```python
from build123d import *

# Parameters (mm, degrees)
SKETCH1_W               = 50
SKETCH1_H               = 50
BOSS_EXTRUDE1_DEPTH     = 2
CUT_EXTRUDE1_DEPTH      = 36.411862419
CUT_EXTRUDE1_DEPTH_BACK = 36.411862419
SKETCH2_W               = 2.3
SKETCH2_H               = 16
SKETCH3_W               = 22
SKETCH3_H               = 3
SKETCH3_W_2             = 5
BOSS_EXTRUDE2_DEPTH     = 14.5
SKETCH4_W               = 5
SKETCH4_H               = 2
SKETCH4_W_2             = 4
BOSS_EXTRUDE11_DEPTH    = 13
SKETCH5_W               = 3.5
SKETCH5_H               = 3
SKETCH5_W_2             = 18
BOSS_EXTRUDE12_DEPTH    = 1
SKETCH6_W               = 3.5
SKETCH6_H               = 12
SKETCH6_W_2             = 3
BOSS_EXTRUDE13_DEPTH    = 9
SKETCH7_W               = 3.5
SKETCH7_H               = 8
BOSS_EXTRUDE14_DEPTH    = 11
SKETCH8_W               = 2
SKETCH8_H               = 8
BOSS_EXTRUDE15_DEPTH    = 8
BOSS_EXTRUDE16_DEPTH    = 20
SKETCH10_W              = 2
SKETCH10_H              = 15
BOSS_EXTRUDE17_DEPTH    = 8
FILLET1_R               = 10
FILLET2_START           = -18
FILLET2_DEPTH           = 0.13972
FILLET2_START_2         = -17.86028
FILLET2_2_DEPTH         = 8.733515347
FILLET2_START_3         = -25
FILLET2_3_DEPTH         = 8.873235347
CUT_EXTRUDE2_DEPTH      = 50.964612469
CUT_EXTRUDE2_DEPTH_BACK = 50.964612469
SKETCH11_R              = 1.65
SKETCH13_W              = 2.5
SKETCH13_H              = 21
BOSS_EXTRUDE18_DEPTH    = 2
FILLET3_R               = 4
SKETCH14_W              = 17.5
SKETCH14_H              = 3
BOSS_EXTRUDE19_DEPTH    = 19.5
FILLET4_R               = 3
SKETCH15_W              = 14.5
SKETCH15_H              = 2
BOSS_EXTRUDE20_DEPTH    = 3
FILLET5_R               = 3
FILLET6_R               = 3


with BuildPart() as part:
    # Sketch1 → Boss-Extrude1 (new body)
    with BuildSketch(Plane.XY):
        Rectangle(SKETCH1_W, SKETCH1_H)
    extrude(amount=BOSS_EXTRUDE1_DEPTH)

    # Sketch2 → Cut-Extrude1 (cut, two sides: drawn at the far end of the back side and taken through both)
    with BuildSketch(Plane.XY.offset(2).offset(-CUT_EXTRUDE1_DEPTH_BACK)):
        with Locations((-19.85, 5.5)):
            Rectangle(SKETCH2_W, SKETCH2_H)
        with Locations((22.95, 5.5)):
            Rectangle(SKETCH2_W, SKETCH2_H)
    extrude(amount=CUT_EXTRUDE1_DEPTH + CUT_EXTRUDE1_DEPTH_BACK, mode=Mode.SUBTRACT)

    # Sketch3 → Boss-Extrude2 (add)
    with BuildSketch(Plane(origin=(0, 0, 0), x_dir=(-1, 0, 0), z_dir=(0, 0, -1))):
        with Locations((-14, -21.5)):
            Rectangle(SKETCH3_W, SKETCH3_H)
        with Locations((22.5, -21.5)):
            Rectangle(SKETCH3_W_2, SKETCH3_H)
    extrude(amount=BOSS_EXTRUDE2_DEPTH)

    # Sketch4 → Boss-Extrude11 (add)
    with BuildSketch(Plane(origin=(0, 0, 0), x_dir=(-1, 0, 0), z_dir=(0, 0, -1))):
        with Locations((3.5, -24)):
            Rectangle(SKETCH4_W, SKETCH4_H)
        with Locations((13.5, -24)):
            Rectangle(SKETCH4_W_2, SKETCH4_H)
    extrude(amount=BOSS_EXTRUDE11_DEPTH)

    # Sketch5 → Boss-Extrude12 (add)
    with BuildSketch(Plane(origin=(0, 0, -14.5), x_dir=(-1, 0, 0), z_dir=(0, 0, -1))):
        with Locations((23.25, -21.5)):
            Rectangle(SKETCH5_W, SKETCH5_H)
        with Locations((-16, -21.5)):
            Rectangle(SKETCH5_W_2, SKETCH5_H)
    extrude(amount=BOSS_EXTRUDE12_DEPTH)

    # Sketch6 → Boss-Extrude13 (add)
    with BuildSketch(Plane(origin=(0, 0, 0), x_dir=(-1, 0, 0), z_dir=(0, 0, -1))):
        with Locations((23.25, -14)):
            Rectangle(SKETCH6_W, SKETCH6_H)
        with Locations((-23.5, -14)):
            Rectangle(SKETCH6_W_2, SKETCH6_H)
    extrude(amount=BOSS_EXTRUDE13_DEPTH)

    # Sketch7 → Boss-Extrude14 (add)
    with BuildSketch(Plane(origin=(0, 0, -9), x_dir=(-1, 0, 0), z_dir=(0, 0, -1))):
        with Locations((23.25, -14)):
            Rectangle(SKETCH7_W, SKETCH7_H)
    extrude(amount=BOSS_EXTRUDE14_DEPTH)

    # Sketch8 → Boss-Extrude15 (add)
    with BuildSketch(Plane.ZY.offset(25)):
        with Locations((-19, -14)):
            Rectangle(SKETCH8_W, SKETCH8_H)
    extrude(amount=BOSS_EXTRUDE15_DEPTH)

    # Sketch9 → Boss-Extrude16 (add)
    with BuildSketch(Plane(origin=(0, 0, 0), x_dir=(-1, 0, 0), z_dir=(0, 0, -1))):
        Polygon((11.748068925, 25), (11.748068925, 23), (23, 23), (23, 15.388525781), (25, 15.388525781), (25, 25), align=None)
    extrude(amount=BOSS_EXTRUDE16_DEPTH)

    # Sketch10 → Boss-Extrude17 (add)
    with BuildSketch(Plane.ZY.offset(25)):
        with Locations((-19, 22.888525781)):
            Rectangle(SKETCH10_W, SKETCH10_H)
    extrude(amount=BOSS_EXTRUDE17_DEPTH)

    # Fillet1
    # the kernel refuses this fillet: 10 mm, written as the material it adds along each edge
    with BuildSketch(Plane(origin=(-25, 25, -20), x_dir=(1, 0, 0), z_dir=(0, 0, 1))) as fillet1_piece_1:
        with BuildLine():
            CenterArc((8.873235347, 10), FILLET1_R, 207.461173358, 62.538826642)
            Line((0, 5.388525781), (0, 0))
            Line((0, 0), (8.873235347, 0))
        make_face()
    extrude(amount=2)

    # Fillet2: read off the stored shape, not the designer's step
    # Fillet2 outline → Fillet2 (add)
    with BuildSketch(Plane.XY.offset(FILLET2_START)):
        with BuildLine():
            Line((-25, 30.388525781), (-25, 25))
            Line((-25, 25), (-16.126764653, 25))
            ThreePointArc((-16.126764653, 25), (-21.317393604, 26.452639525), (-25, 30.388525781))
        make_face()
    extrude(amount=FILLET2_DEPTH)

    # Fillet2 2 outline → Fillet2 2 (add)
    with BuildSketch(Plane.XY.offset(FILLET2_START_2)):
        with BuildLine():
            Line((-25, 30.388525781), (-25, 25))
            Line((-25, 25), (-16.126764653, 25))
            ThreePointArc((-16.126764653, 25), (-21.317393604, 26.452639525), (-25, 30.388525781))
        make_face()
    extrude(amount=FILLET2_2_DEPTH)

    # Fillet2 3 outline → Fillet2 3 (cut)
    with BuildSketch(Plane.YZ.offset(FILLET2_START_3)):
        with BuildLine():
            ThreePointArc((25, -9.126764653), (26.452639525, -14.317393604), (30.388525781, -18))
            Line((30.388525781, -18), (32, -18.837492924))
            Line((32, -18.837492924), (32, -9.126764653))
            Line((32, -9.126764653), (25, -9.126764653))
        make_face()
    extrude(amount=FILLET2_3_DEPTH, mode=Mode.SUBTRACT)

    # Sketch11 → Cut-Extrude2 (cut, two sides: drawn at the far end of the back side and taken through both)
    with BuildSketch(Plane(origin=(0, 0, -20), x_dir=(-1, 0, 0), z_dir=(0, 0, -1)).offset(-CUT_EXTRUDE2_DEPTH_BACK)):
        with Locations((28.55, 26)):
            Circle(SKETCH11_R)
        with Locations((28.55, -14)):
            Circle(SKETCH11_R)
    extrude(amount=CUT_EXTRUDE2_DEPTH + CUT_EXTRUDE2_DEPTH_BACK, mode=Mode.SUBTRACT)

    # Sketch13 → Boss-Extrude18 (add)
    with BuildSketch(Plane(origin=(0, 0, 0), x_dir=(-1, 0, 0), z_dir=(0, 0, -1))):
        with Locations((-26.25, 5.5)):
            Rectangle(SKETCH13_W, SKETCH13_H)
    extrude(amount=-BOSS_EXTRUDE18_DEPTH)

    # Fillet3
    # the kernel refuses this fillet: 4 mm, written as the material it adds along each edge
    with BuildSketch(Plane(origin=(25, -5, -9.270248109), x_dir=(0, -1, 0), z_dir=(0, 0, 1))) as fillet3_piece_1_section:
        with BuildLine():
            CenterArc((3.708099244, 4), FILLET3_R, 202.024312837, 67.975687163)
            Line((0, 2.5), (-0.074161985, 2.47))
            ThreePointArc((-0.074161985, 2.47), (-0.08, 1.25), (-0.08, 0))
            Line((-0.08, 0), (0, -0.08))
            Line((0, -0.08), (3.708099244, -0.08))
            Line((3.708099244, -0.08), (3.708099244, 0))
        make_face()
    fillet3_piece_1 = extrude(amount=11.270248109, mode=Mode.PRIVATE)
    fillet3_piece_1 = split(fillet3_piece_1, bisect_by=Plane(origin=(25, -5, 0), z_dir=(0, 0, -1)), keep=Keep.TOP, mode=Mode.PRIVATE)
    fillet3_piece_1 = split(fillet3_piece_1, bisect_by=Plane(origin=(25, -8, -9.270248109), z_dir=(0, -1, 0)), keep=Keep.TOP, mode=Mode.PRIVATE)
    fillet3_piece_1 = split(fillet3_piece_1, bisect_by=Plane(origin=(25, -5, -9), z_dir=(0, 0, 1)), keep=Keep.TOP, mode=Mode.PRIVATE)
    add(fillet3_piece_1)
    with BuildSketch(Plane(origin=(25, -5, 0), x_dir=(0, -1, 0), z_dir=(0, 0, 1))) as fillet3_piece_2_section:
        with BuildLine():
            CenterArc((3.708099244, 4), FILLET3_R, 202.024312837, 67.975687163)
            Line((0, 2.5), (-0.074161985, 2.47))
            ThreePointArc((-0.074161985, 2.47), (-0.08, 1.25), (-0.08, 0))
            Line((-0.08, 0), (0, -0.08))
            Line((0, -0.08), (3.708099244, -0.08))
            Line((3.708099244, -0.08), (3.708099244, 0))
        make_face()
    fillet3_piece_2 = extrude(amount=2, mode=Mode.PRIVATE)
    fillet3_piece_2 = split(fillet3_piece_2, bisect_by=Plane(origin=(25, -8, 0), z_dir=(0, -1, 0)), keep=Keep.TOP, mode=Mode.PRIVATE)
    add(fillet3_piece_2)
    with BuildSketch(Plane(origin=(25, -5, 0), x_dir=(0, -1, 0), z_dir=(0, 0, 1))) as fillet3_piece_3_section:
        with BuildLine():
            CenterArc((3.708099244, 4), FILLET3_R, 202.024312837, 67.975687163)
            Line((0, 2.5), (-0.074161985, 2.47))
            ThreePointArc((-0.074161985, 2.47), (-0.08, 1.25), (-0.08, 0))
            Line((-0.08, 0), (0, -0.08))
            Line((0, -0.08), (3.708099244, -0.08))
            Line((3.708099244, -0.08), (3.708099244, 0))
        make_face()
    fillet3_piece_3 = extrude(amount=2, mode=Mode.PRIVATE)
    fillet3_piece_3 = split(fillet3_piece_3, bisect_by=Plane(origin=(25, -8, 0), z_dir=(0, 1, 0)), keep=Keep.TOP, mode=Mode.PRIVATE)
    add(fillet3_piece_3)
    with BuildSketch(Plane(origin=(25, 16, 0), x_dir=(0, 1, 0), z_dir=(0, 0, 1))) as fillet3_piece_4:
        with BuildLine():
            CenterArc((3.708099244, -4), FILLET3_R, 90, 67.975687163)
            Line((0, -2.5), (-0.074161985, -2.47))
            ThreePointArc((-0.074161985, -2.47), (-0.08, -1.25), (-0.08, 0))
            Line((-0.08, 0), (0, 0.08))
            Line((0, 0.08), (3.708099244, 0.08))
            Line((3.708099244, 0.08), (3.708099244, 0))
        make_face()
    extrude(amount=2)

    # Sketch14 → Boss-Extrude19 (add)
    with BuildSketch(Plane(origin=(0, 0, 0), x_dir=(-1, 0, 0), z_dir=(0, 0, -1))):
        with Locations((-13.25, -17.4)):
            Rectangle(SKETCH14_W, SKETCH14_H)
    extrude(amount=BOSS_EXTRUDE19_DEPTH)

    # Fillet4
    fillet4_edges = [part.edges().sort_by_distance(p)[0] for p in [
        (-3.5, -23, 0),
        (-13.5, -23, 0),
    ]]
    fillet(fillet4_edges, radius=FILLET4_R)

    # Sketch15 → Boss-Extrude20 (add)
    with BuildSketch(Plane.XZ.offset(25)):
        with Locations((-8.25, 1)):
            Rectangle(SKETCH15_W, SKETCH15_H)
    extrude(amount=BOSS_EXTRUDE20_DEPTH)

    # Fillet5
    # the kernel refuses this fillet: 3 mm, written as the material it adds along each edge
    with BuildSketch(Plane(origin=(-15.5, -25, 2), x_dir=(-1, 0, 0), z_dir=(0, 0, -1)), Plane(origin=(-1, -25, 0), x_dir=(1, 0, 0), z_dir=(0, 0, 1))) as fillet5_piece_1:
        with BuildLine():
            CenterArc((FILLET5_R, -FILLET5_R), FILLET5_R, 90, 90)
            Line((0, -FILLET5_R), (0, 0))
            Line((0, 0), (FILLET5_R, 0))
        make_face()
    extrude(amount=2)

    # Fillet6
    fillet6_edges = [part.edges().sort_by_distance(p)[0] for p in [
        (-3.5, -25, 0),
        (-13.5, -25, 0),
    ]]
    fillet(fillet6_edges, radius=FILLET6_R - 0.0001)  # a hair under: the kernel refuses the full size


solid = part.part
```
Can you work these out from the model? Positions are in its coordinate system, mm. A direction names the side the tool comes from. Give positions to 0.01 mm unless a question says otherwise; leave off trailing zeros. Loops run counter-clockwise (first coordinate to the right, second up) from the corner with the lowest first, then second, coordinate; pieces in that order, holes last. Notation, with made-up numbers: M 15,64 L 33,64 A17 cw 33,79 Z; hole C 35.25,46.5 d7. An arc over 180 degrees is marked long. One line per item, written item: value.
(1) Suppose I cut it at B-B on x = -28.55. List the corners of the cut face in (y, z) for me.
Returned:
outline: M -18,-20 L -15.65,-20 L -15.65,-18 L -18,-18 Z; M -12.35,-20 L -10,-20 L -10,-18 L -12.35,-18 Z; M 15.39,-20 L 24.35,-20 L 24.35,-18 L 15.39,-18 Z; M 27.65,-20 L 30.39,-20 L 30.39,-18 L 27.65,-18 Z
(2) Suppose I cut it at C-C on y = -14. List the corners of the cut face in (x, z) for me.
Returned:
outline: M -33,-20 L -30.2,-20 L -30.2,-18 L -33,-18 Z; M -26.9,-20 L -21.5,-20 L -21.5,0 L 22,0 L 22,-9 L 25,-9 L 25,2 L -25,2 L -25,-18 L -26.9,-18 Z
(3) I need wall thicknesses on line 1 (Y direction, x = -28.55, z = -19.25); line 2 (Y direction, x = 5.5, z = -14.25); line 3 (X direction, y = -14, z = -18.7). Which ranges of each line are inside material? Lowest first, please.
Returned:
line 1: -18 to -15.65, -12.35 to -10, 15.39 to 24.35, 27.65 to 30.39
line 2: -23 to -20, -18.9 to -15.9
line 3: -33 to -30.2, -26.9 to -21.5
(4) Which directions (+Z, -Z, +X, -X, +Y, -Y) give clear straight access to the entire face, cutting with the end or side of a thin tool? Please do faces 1 (the face through (-4, -25, -8)), 2 (the face through (-21, -21, -14.5)), 3 (the face through (24, -8, -4)), 4 (the face through (-22, -25, 1)), 5 (the face through (-11.748, 24, -10)).
Returned:
face 1: -Z, +X, -X, -Y
face 2: -Z, -Y
face 3: -Z, +X, -X, +Y
face 4: +Z, -Z, -X, -Y
face 5: -Z, +X, +Y
(5) Suppose I cut it at A-A on z = -7.25. Count the separate pieces of the cut face and the enclosed holes in it, plus the area to 3 significant figures.
Returned:
separate pieces: 5
enclosed holes: 0
area: 271 mm^2
(6) Will these pins go through, and if not, where does the flat tip stop? pin 1 (1.5 mm diameter, centred on y = -21.5, z = -9.5, fed in from +X); pin 2 (2.5 mm diameter, centred on x = 24, y = -16, fed in from -Z); pin 3 (1.6 mm diameter, centred on x = -2.5, y = -23.5, fed in from -Z).
Returned:
pin 1: x = 25
pin 2: z = -9
pin 3: z = -13
(7) We'd pull the mould along Y, two halves only. Please class faces 6 (the face through (-29, 23, -18)), 7 (the face through (-3.46, -25.9, -0.86)), 8 (the face through (-21.5, -14, -10)): released by +Y, released by -Y, zero draft, split by the parting line, or undercut.
Returned:
face 6: zero draft
face 7: released by -Y
face 8: undercut
